Geometry: see drawing. Coordinates: mm, zero at the bounding-box minimum. A direction names the side the tool comes from. Coordinates: 2 decimals unless noted, no trailing zeros. Order: outer loops, then holes, each group sorted by start corner. A loop starts at its lowest first (then second) coordinate and runs counter-clockwise, first axis right, second up.
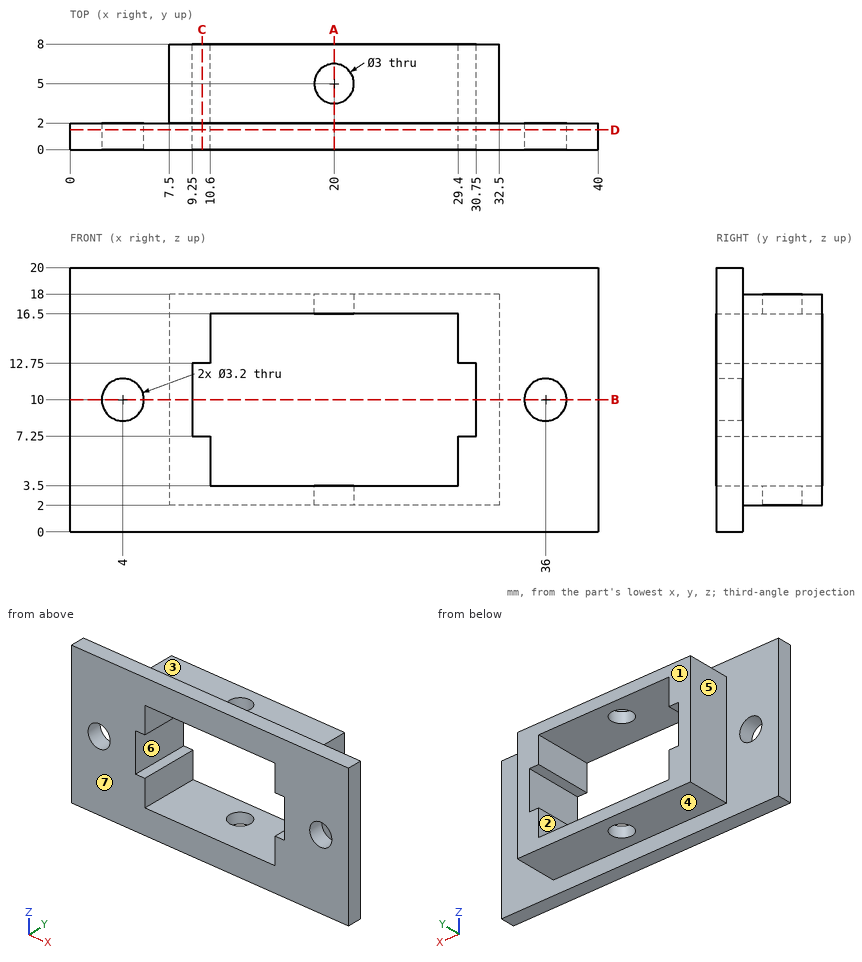
Item 1: Cut plane A-A on x = 20. Return loops of the section in (y, z), then the cut area to 3 significant figures.
Response values:
outline: (0, 0) - (2, 0) - (2, 2) - (3.5, 2) - (3.5, 3.5) - (0, 3.5) - close; (0, 16.5) - (3.5, 16.5) - (3.5, 18) - (2, 18) - (2, 20) - (0, 20) - close; (6.5, 2) - (8, 2) - (8, 3.5) - (6.5, 3.5) - close; (6.5, 16.5) - (8, 16.5) - (8, 18) - (6.5, 18) - close
area: 23.0 mm2
Item 2: Cut plane B-B on z = 10. Return loops of the section in (x, y).
Response values:
outline: (0, 0) - (2.4, 0) - (2.4, 2) - (0, 2) - close; (5.6, 0) - (9.25, 0) - (9.25, 8) - (7.5, 8) - (7.5, 2) - (5.6, 2) - close; (30.75, 0) - (34.4, 0) - (34.4, 2) - (32.5, 2) - (32.5, 8) - (30.75, 8) - close; (37.6, 0) - (40, 0) - (40, 2) - (37.6, 2) - close
Item 3: Access query for the marked faces 5, 6 and 7. Directions: +Z, -Z, +X, -X, +Y, -Y. A direction counts if a zero-diameter tool reaches every point of the face in a straight line with its end or side. Return the directions, or none.
Response values:
face 5: +Z, -Z, -X, +Y
face 6: +Y, -Y
face 7: +Z, -Z, +X, -X, -Y
Item 4: Cut plane C-C on x = 10. Return loops of the section in (y, z).
Response values:
outline: (0, 0) - (2, 0) - (2, 2) - (8, 2) - (8, 7.25) - (0, 7.25) - close; (0, 12.75) - (8, 12.75) - (8, 18) - (2, 18) - (2, 20) - (0, 20) - close
Item 5: Pin query (flat end, axial travel): pin 1 Ø1.5 at (y, z) = (3, 2) entering from -X; pin 2 Ø3 at (y, z) = (5.5, 11.5) entering from +X; pin 3 Ø4 at (x, y) = (20, 5) entering from -Z. Return the tip coordinate at first contact, or that it passes through.
Response values:
pin 1: stops at x = 7.5
pin 2: stops at x = 32.5
pin 3: stops at z = 2
Item 6: Cut plane D-D on y = 1.5. Return loops of the section in (x, z), then the cut area to 3 significant figures.
Response values:
outline: (0, 0) - (40, 0) - (40, 20) - (0, 20) - close; hole circle Ø3.2 at (4, 10); hole (9.25, 7.25) - (10.6, 7.25) - (10.6, 3.5) - (29.4, 3.5) - (29.4, 7.25) - (30.75, 7.25) - (30.75, 12.75) - (29.4, 12.75) - (29.4, 16.5) - (10.6, 16.5) - (10.6, 12.75) - (9.25, 12.75) - close; hole circle Ø3.2 at (36, 10)
area: 525 mm2
Item 7: Ray query, probe 1 along Z at (x, y) = (19, 3.75); probe 2 along X at (y, z) = (3.25, 7.5); probe 3 along Z at (x, y) = (29.5, 3). Return the intervals inside material, ascending.
Response values:
probe 1: z = 2 to 3.5, 16.5 to 18
probe 2: x = 7.5 to 9.25, 30.75 to 32.5
probe 3: z = 2 to 7.25, 12.75 to 18
Item 8: Draft query along Z for the marked faces 1, 2, 3 and 4. Return one class per face: pulls with the +Z half, pulls with the -Z half, needs draft (parallel to the pull), parting line crosses it, or undercut.
Response values:
face 1: needs draft
face 2: undercut
face 3: pulls with the +Z half
face 4: pulls with the -Z half
